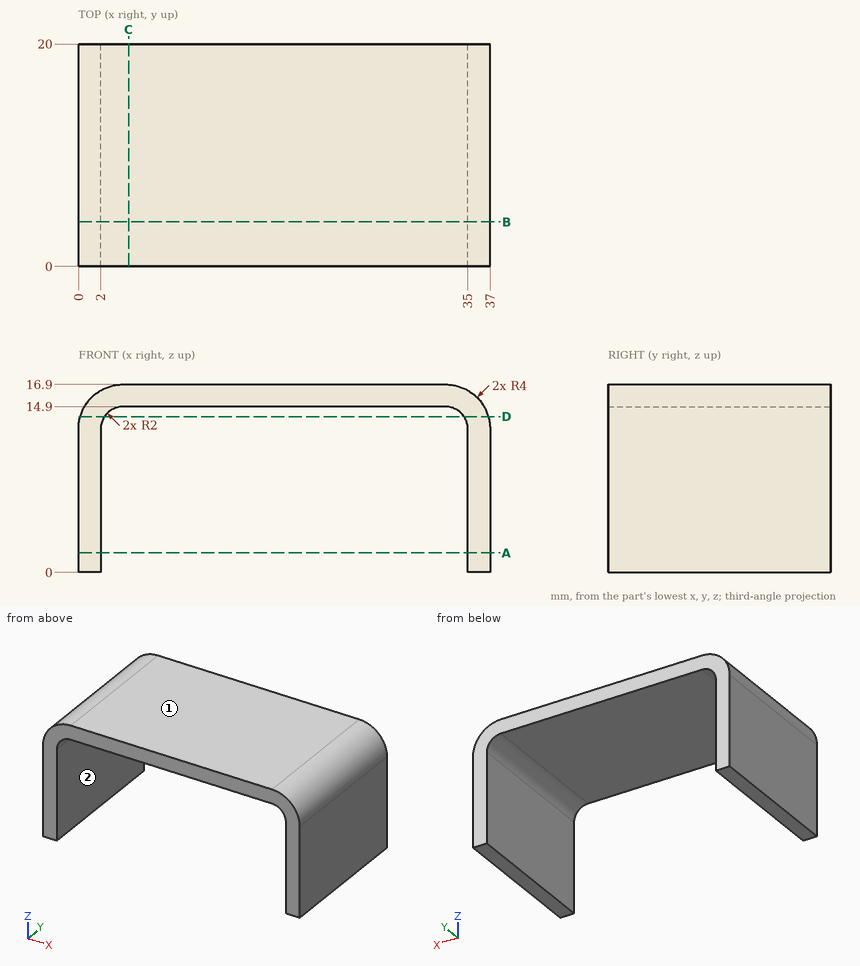
Source: three-view drawing plus pictorial views. Frame: mm from the lowest corner of the part. A direction names the side the tool comes from. Coordinates: 2 decimals unless noted, no trailing zeros. Order: outer loops, then holes, each group sorted by start corner. A loop starts at its lowest first (then second) coordinate and runs counter-clockwise, first axis right, second up. Notation, with made-up numbers: M 82,58.25 L 117,58.25 A19 cw 117,95.25 Z; hole C 42.5,2.5 d6. An arc over 180 degrees is marked long. Answer in a Markdown table with one row per item.
(1) Section query C-C, the plane x = 4.5. Output: boundary loops of the cut face in (y, z), plus the area to 3 significant figures.
Numbers:
| item | result |
|---|---|
| outline | M 0,14.9 L 20,14.9 L 20,16.9 L 0,16.9 Z |
| area | 40.0 mm^2 |
(2) Contact query for flat-ended pins moving along their axis: pin 1 Ø5 at (x, y) = (33, 3.5) entering from -Z; pin 2 Ø4 at (x, y) = (12.5, 15.5) entering from -Z. Output: stop coordinate, or through.
Numbers:
| item | result |
|---|---|
| pin 1 | stops at z = 0 |
| pin 2 | stops at z = 14.9 |
(3) Section query B-B, the plane y = 4. Output: boundary loops of the cut face in (x, z), plus the area to 3 significant figures.
Numbers:
| item | result |
|---|---|
| outline | M 0,0 L 2,0 L 2,12.9 A2 cw 4,14.9 L 33,14.9 A2 cw 35,12.9 L 35,0 L 37,0 L 37,12.9 A4 ccw 33,16.9 L 4,16.9 A4 ccw 0,12.9 Z |
| area | 128 mm^2 |
(4) Access query for the marked faces 1 and 2. Directions: +Z, -Z, +X, -X, +Y, -Y. A direction counts if a zero-diameter tool reaches every point of the face in a straight line with its end or side. Return the directions, or none.
Numbers:
| item | result |
|---|---|
| face 1 | +Z, +X, -X, +Y, -Y |
| face 2 | -Z, +Y, -Y |
(5) Section query D-D, the plane z = 14. Output: boundary loops of the cut face in (x, y).
Numbers:
| item | result |
|---|---|
| outline | M 0.15,0 L 2.33,0 L 2.33,20 L 0.15,20 Z; M 34.67,0 L 36.85,0 L 36.85,20 L 34.67,20 Z |
(6) Material intervals for line 1 (X direction, y = 7, z = 11); line 2 (Z direction, x = 12.5, y = 4.25); line 3 (Z direction, x = 33.5, y = 14.75), sorted ascending. Write a range as [from, to].
Numbers:
| item | result |
|---|---|
| line 1 | x = [0, 2], [35, 37] |
| line 2 | z = [14.9, 16.9] |
| line 3 | z = [14.84, 16.87] |
(7) Section query A-A, the plane z = 1.75. Output: boundary loops of the cut face in (x, y).
Numbers:
| item | result |
|---|---|
| outline | M 0,0 L 2,0 L 2,20 L 0,20 Z; M 35,0 L 37,0 L 37,20 L 35,20 Z |
